```python
from build123d import *

# Parameters (mm, degrees)
F1_DEPTH = 101.6
F2_R     = 6.35
F3_SIZE2 = 5.08
F3_SIZE  = 5.08
F4_SIZE2 = 5.08
F4_SIZE  = 5.08
F5_R     = 6.35


with BuildPart() as f1:
    # F0 (on Top) → F1 (new body)
    with BuildSketch(Plane.XY):
        Polygon((-52.913923, 29.352266), (-122.807145, 29.352266), (-122.807145, 11.568784), (-91.789439, 11.568784), (-91.789439, -9.523253), (-121.566437, -9.523253), (-121.566437, -26.066026), (-52.913923, -26.066026), (0, 0), align=None)
    extrude(amount=F1_DEPTH)

    # F2
    f2_edges = [f1.edges().sort_by_distance(p)[0] for p in [
        (-121.566437, -26.066026, 50.8),
        (-122.807145, 29.352266, 50.8),
    ]]
    fillet(f2_edges, radius=F2_R)

    # F3
    f3_edges = [f1.edges().sort_by_distance(p)[0] for p in [
        (-91.789439, 11.568784, 50.8),
    ]]
    chamfer(f3_edges, length=F3_SIZE, length2=F3_SIZE2)

    # F4
    f4_edges = [f1.edges().sort_by_distance(p)[0] for p in [
        (-91.789439, -9.523253, 50.8),
    ]]
    chamfer(f4_edges, length=F4_SIZE, length2=F4_SIZE2)

    # F5
    f5_edges = [f1.edges().sort_by_distance(p)[0] for p in [
        (0, 0, 50.8),
    ]]
    fillet(f5_edges, radius=F5_R)


solid = f1.part
```
Work out the finished part from the listing and answer in its coordinate system (mm). A direction names the side the tool comes from. Coordinates: 2 decimals unless noted, no trailing zeros. Loops run counter-clockwise (first coordinate to the right, second up) from the corner with the lowest first, then second, coordinate; pieces in that order, holes last.
1) Section B-B (z = 94) is taken. Give the vertices of the cut face in (x, y).
Results:
outline: (-122.81, 11.57) - (-96.87, 11.57) - (-91.79, 6.49) - (-91.79, -4.44) - (-96.87, -9.52) - (-121.57, -9.52) - (-121.57, -19.72) arc R6.35 ccw to (-115.22, -26.07) - (-52.91, -26.07) - (-10.89, -5.36) arc R6.35 ccw to (-10.61, 5.89) - (-52.91, 29.35) - (-116.46, 29.35) arc R6.35 ccw to (-122.81, 23) - close
2) Section A-A (x = -108) is taken. Give the vertices of the cut face in (y, z).
Results:
outline: (-26.07, 0) - (-9.52, 0) - (-9.52, 101.6) - (-26.07, 101.6) - close; (11.57, 0) - (29.35, 0) - (29.35, 101.6) - (11.57, 101.6) - close
3) Section D-D (x = -25.5) is taken. Give the vertices of the cut face in (y, z), plus the area to 3 significant figures.
Results:
outline: (-12.56, 0) - (14.15, 0) - (14.15, 101.6) - (-12.56, 101.6) - close
area: 2,710 mm2
4) Flat-ended cylindrical pins translate along their axes: pin 1 (8 mm diameter, centred on x = -48, z = 50.5, fed in from -Y); pin 2 (6 mm diameter, centred on y = -19.5, z = 44, fed in from +X); pin 3 (5.5 mm diameter, centred on y = 3, z = 46.5, fed in from -X). Find the tip coordinate at first contact, or state that the pin passes through.
Results:
pin 1: stops at y = -25.62
pin 2: stops at x = -33.49
pin 3: stops at x = -91.79
5) Consider probe 1 along Y at (x, z) = (-108.5, 8); probe 2 along X at (y, z) = (23, 82.5); probe 3 along X at (y, z) = (15.5, 20). Determine where each line is inside the solid, lowest interval first.
Results:
probe 1: y = -26.07 to -9.52, 11.57 to 29.35
probe 2: x = -122.81 to -41.46
probe 3: x = -122.81 to -27.94
6) For a pull along Y with two mould halves and no side action, classify faces 4 (the flat face through (-32.194, -15.859, 50.089)), 5 (the flat face through (-66, 2, 101.6)), 6 (the flat face through (-94.365, -7.019, 50.089)) as +Y half, -Y half, draft (parallel to the pull), parting line (faces both ways), or undercut.
Results:
face 4: -Y half
face 5: draft
face 6: undercut
7) For faces 1 (the flat face through (-121.566, -15, 50)), 2 (the flat face through (-110, 11.569, 50)), 3 (the cylindrical face through (-120.9, 27.54, 51.51)), determine the directions among +Z, -Z, +X, -X, +Y, -Y from which every point of the face is accessible in a straight line to the end or side of a thin tool.
Results:
face 1: +Z, -Z, -X, -Y
face 2: +Z, -Z, -X
face 3: +Z, -Z, -X, +Y
8) Section C-C (y = -14) is taken. Give the vertices of the cut face in (x, z).
Results:
outline: (-121.57, 0) - (-28.42, 0) - (-28.42, 101.6) - (-121.57, 101.6) - close
